Autodesk Fusion 360 part; units mm, degrees
sketch "Sketch1" plane through (0, 0, 0) normal (0, 1, 0) x (1, 0, 0)
  line L0 (43, -28.5) -> (-43, -28.5)
  line L1 (-43, -28.5) -> (-43, 28.5)
  line L2 (-43, 28.5) -> (43, 28.5)
  line L3 (43, 28.5) -> (43, -28.5)
  line L4 (43, -28.5) -> (-43, 28.5) construction
  line L5 (-43, -28.5) -> (43, 28.5) construction
  line L6 (43, -28.5) -> (39, -28.5)
  line L7 (39, -28.5) -> (39, -24.5)
  line L8 (39, -24.5) -> (43, -24.5)
  line L9 (43, -24.5) -> (43, -28.5)
  circle A0 centre (39, -24.5) radius 2.5
  line L10 (52.3114, 0) -> (-55.6196, 0)
  line L11 (0, 36.5366) -> (0, -32.8551)
  circle A1 centre (-39, -24.5) radius 2.5
  circle A2 centre (39, 24.5) radius 2.5
  circle A3 centre (-39, 24.5) radius 2.5
  dimension "d1" = 86
  dimension "d2" = 57
  dimension "d5" = 4
  dimension "d6" = 4
  dimension "d7" = 5
extrude "Extrude1" add sketch "Sketch1" along normal blind 9 contours L0 L3 L6 L7 L8 L9 A0 | L0 L3 L7 L8 A0 L10 L11 | L0 L1 L10 L11 | L7 L8 A0 | L7 L8 A0 | L2 L3 L10 L11 | L1 L2 L10 L11 | A1 | A2 | A3
extrude "Extrude2" add sketch "Sketch1" along normal blind 25 contours L7 L8 A0 | L7 L8 A0 | A1 | A2 | A3
Read the model definition and answer for the solid it produces. Units are mm, in the model's axes. A direction names the side the tool comes from. Coordinates: 2 decimals unless noted, no trailing zeros. Order: outer loops, then holes, each group sorted by start corner. A loop starts at its lowest first (then second) coordinate and runs counter-clockwise, first axis right, second up. Notation, with made-up numbers: (-11.75, 85) - (-2.75, 85) arc R28 cw to (-2.75, 109) - close; hole circle Ø11 at (74.5, 86.25). An arc over 180 degrees is marked (long way). Use one line per item in the form item = value.
(1) Given pin 1 Ø12 at (x, y) = (-11.5, 16) entering from -Z; pin 2 Ø4 at (x, z) = (12, -18) entering from +Y, each flat-ended and moving along its own axis, determine where each tip first touches the part or whether it passes through.
Computed values:
pin_1 = through
pin_2 = 9
(2) Section D-D, the plane z = -6 is taken. Give the vertices of the cut face in (x, y), then the cut area to 3 significant figures.
Computed values:
outline = (-43, 0) - (43, 0) - (43, 9) - (-43, 9) - close
area = 774 mm²
(3) Section B-B, the plane x = 39 is taken. Give the vertices of the cut face in (y, z), then the cut area to 3 significant figures.
Computed values:
outline = (0, -28.5) - (9, -28.5) - (9, -27) - (25, -27) - (25, -22) - (9, -22) - (9, 22) - (25, 22) - (25, 27) - (9, 27) - (9, 28.5) - (0, 28.5) - close
area = 673 mm²
(4) Section A-A, the plane z = -24.5 is taken. Give the vertices of the cut face in (x, y), then the cut area to 3 significant figures.
Computed values:
outline = (-43, 0) - (43, 0) - (43, 9) - (41.5, 9) - (41.5, 25) - (36.5, 25) - (36.5, 9) - (-36.5, 9) - (-36.5, 25) - (-41.5, 25) - (-41.5, 9) - (-43, 9) - close
area = 934 mm²
(5) Which of the six approach directions +Z, -Z, +X, -X, +Y, -Y give full straight-line access (tool end or side, diameter ignored) to faces 4 (the face through (-1, 9, 0)), 5 (the face through (-1, 0, 0))?
Computed values:
face_4 = +Y
face_5 = +Z, -Z, +X, -X, -Y
(6) Straight lines are drawn through the part: L1, parallel to Y at x = 3, z = -3; L2, parallel to Z at x = 39, y = 21.75; L3, parallel to X at y = 18.25, z = -24. For each, find the intervals that lie inside material, in ascending order.
Computed values:
L1 = 0 to 9
L2 = -27 to -22, 22 to 27
L3 = -41.45 to -36.55, 36.55 to 41.45
(7) For a pull along Z with two mould halves and no side action, classify faces 1 (the face through (-39, 25, -25)), 2 (the face through (1, 4, 28.5)), 3 (the face through (-37.66, 16.89, -22.39)) as pulls with the +Z half, pulls with the -Z half, needs draft (parallel to the pull), parting line crosses it, or undercut.
Computed values:
face_1 = needs draft
face_2 = pulls with the +Z half
face_3 = undercut
(8) Section C-C, the plane y = 16.5 is taken. Give the vertices of the cut face in (x, z), then the cut area to 3 significant figures.
Computed values:
outline = circle Ø5 at (-39, -24.5); circle Ø5 at (-39, 24.5); circle Ø5 at (39, -24.5); circle Ø5 at (39, 24.5)
area = 78.5 mm²
